The listing builds one solid part. Answer for the finished solid, in the listing's coordinates (mm). A direction names the side the tool comes from. Round coordinates to 2 decimals unless told otherwise and drop trailing zeros. Loops run counter-clockwise (first coordinate to the right, second up) from the corner with the lowest first, then second, coordinate; pieces in that order, holes last. Notation, with made-up numbers: (40.5, 81) - (52.5, 81) arc R24 cw to (52.5, 117) - close; hole circle Ø7 at (51, 58.5). An arc over 180 degrees is marked (long way). One line per item, written item: value.
```python
from build123d import *

# Parameters (mm, degrees)
SKETCH1_W           = 51
SKETCH1_H           = 82
SKETCH1_R           = 1.6
BOSS_EXTRUDE1_DEPTH = 22
SKETCH1_3_W         = 10
SKETCH1_3_H         = 15
BOSS_EXTRUDE2_DEPTH = 15
FILLET1_R           = 5


with BuildPart() as part:
    # Sketch1 → Boss-Extrude1 (new body)
    with BuildSketch(Plane(origin=(0, 0, 0), x_dir=(1, 0, 0), z_dir=(0, 1, 0))):
        Rectangle(SKETCH1_W, SKETCH1_H)
        with Locations(Location((0, -37.1, 0), (0, 0, 270))):
            Circle(SKETCH1_R, mode=Mode.SUBTRACT)
        with Locations(Location((0, 37.1, 0), (0, 0, 270))):
            Circle(SKETCH1_R, mode=Mode.SUBTRACT)
    extrude(amount=BOSS_EXTRUDE1_DEPTH)

    # Sketch1_3 → Boss-Extrude2 (add)
    with BuildSketch(Plane(origin=(0, 0, 0), x_dir=(1, 0, 0), z_dir=(0, 1, 0))):
        with Locations((-30.5, -10.5)):
            Rectangle(SKETCH1_3_W, SKETCH1_3_H)
    extrude(amount=BOSS_EXTRUDE2_DEPTH)

    # Fillet1
    fillet1_edges = [part.edges().sort_by_distance(p)[0] for p in [
        (-25.5, 11, 41),
        (-25.5, 11, -41),
        (25.5, 11, -41),
        (25.5, 11, 41),
    ]]
    fillet(fillet1_edges, radius=FILLET1_R)


solid = part.part
```
1) A cutting plane is placed at A-A on x = 0. Give the vertices of the cut face in (y, z), and give its area (3 significant figures).
Final values:
outline: (0, -41) - (22, -41) - (22, -38.7) - (0, -38.7) - close; (0, -35.5) - (22, -35.5) - (22, 35.5) - (0, 35.5) - close; (0, 38.7) - (22, 38.7) - (22, 41) - (0, 41) - close
area: 1,660 mm2
2) For faces 1 (the flat face through (0, 11, 41)), 2 (the flat face through (-31, 15, 10)), 3 (the flat face through (-31, 7, 3)), 4 (the flat face through (-31, 7, 18)), determine the directions among +Z, -Z, +X, -X, +Y, -Y from which every point of the face is accessible in a straight line to the end or side of a thin tool.
Final values:
face 1: +Z, +X, -X, +Y, -Y
face 2: +Z, -Z, -X, +Y
face 3: -Z, -X, +Y, -Y
face 4: +Z, -X, +Y, -Y
3) A cutting plane is placed at C-C on z = 37.1. Give the vertices of the cut face in (x, y).
Final values:
outline: (-25.38, 0) - (-1.6, 0) - (-1.6, 22) - (-25.38, 22) - close; (1.6, 0) - (25.38, 0) - (25.38, 22) - (1.6, 22) - close
4) A cutting plane is placed at B-B on y = 19.5. Give the vertices of the cut face in (x, z), and give its area (3 significant figures).
Final values:
outline: (-25.5, -36) arc R5 ccw to (-20.5, -41) - (20.5, -41) arc R5 ccw to (25.5, -36) - (25.5, 36) arc R5 ccw to (20.5, 41) - (-20.5, 41) arc R5 ccw to (-25.5, 36) - close; hole circle Ø3.2 at (0, -37.1); hole circle Ø3.2 at (0, 37.1)
area: 4,140 mm2
5) A cutting plane is placed at D-D on y = 7.5. Give the vertices of the cut face in (x, z).
Final values:
outline: (-35.5, 3) - (-25.5, 3) - (-25.5, -36) arc R5 ccw to (-20.5, -41) - (20.5, -41) arc R5 ccw to (25.5, -36) - (25.5, 36) arc R5 ccw to (20.5, 41) - (-20.5, 41) arc R5 ccw to (-25.5, 36) - (-25.5, 18) - (-35.5, 18) - close; hole circle Ø3.2 at (0, -37.1); hole circle Ø3.2 at (0, 37.1)
6) Each of these flat-tipped pins is pushed along its axis until it touches: pin 1 Ø1.5 at (y, z) = (19, 17.5) entering from -X; pin 2 Ø11 at (x, y) = (-33, 5) entering from +Z. Where does it stop, or does it pass through?
Final values:
pin 1: x = -25.5
pin 2: z = 18
7) Consider L1, parallel to X at y = 10.5, z = 22.5; L2, parallel to X at y = 6.75, z = 37; L3, parallel to Z at x = 21, y = 19.25. Determine where each line is inside the solid, lowest interval first.
Final values:
L1: -25.5 to 25.5
L2: -25.4 to -1.6, 1.6 to 25.4
L3: -40.97 to 40.97
8) For a pull along X with two mould halves and no side action, classify faces 5 (the flat face through (1, 0, -1)), 6 (the cylindrical face through (0.07, 10.85, -38.7)), 7 (the flat face through (25.5, 11, 1)) as released by +X, released by -X, zero draft, split by the parting line, or undercut.
Final values:
face 5: zero draft
face 6: undercut
face 7: released by +X
